from build123d import *

# Parameters (mm, degrees)
F0_R     = 25
F0_W     = 17
F0_H     = 7
F1_DEPTH = 18
F3_D     = 10
F3_DEPTH = 100
F3_TIP   = 3.0043030951
F4_W     = 17
F4_H     = 1
F5_DEPTH = 2
F6_W     = 3.5
F6_H     = 1
F7_DEPTH = 2


with BuildPart() as f1:
    # F0 (on Top) → F1 (new body)
    with BuildSketch(Plane.XY):
        Circle(F0_R)
        Rectangle(F0_W, F0_H, mode=Mode.SUBTRACT)
    extrude(amount=F1_DEPTH)

    # F3 (one way)
    with BuildSketch(Plane(origin=(0, -3.5, 0), x_dir=(-1, 0, 0), z_dir=(0, -1, 0))):
        with Locations((0, 0)):
            Circle(F3_D / 2)
    extrude(amount=-F3_DEPTH, mode=Mode.SUBTRACT)
    with Locations(Plane(origin=(0, -3.5, 0), x_dir=(-1, 0, 0), z_dir=(0, -1, 0))):
        with Locations((0, 0)):
            with Locations((0, 0, -(F3_DEPTH + F3_TIP / 2))):  # 118° drill point
                Cone(0, F3_D / 2, F3_TIP, mode=Mode.SUBTRACT)

    # F4 (on face) → F5 (join)
    with BuildSketch(Plane(origin=(0, -3.5, 0), x_dir=(-1, 0, 0), z_dir=(0, 1, 0))):
        with Locations((0, 0.5)):
            Rectangle(F4_W, F4_H)
    extrude(amount=F5_DEPTH)

    # F6 (on face) → F7 (join)
    with BuildSketch(Plane.XZ.offset(-3.5)):
        with Locations((-6.75, 0.5)):
            Rectangle(F6_W, F6_H)
        with Locations((6.75, 0.5)):
            Rectangle(F6_W, F6_H)
    extrude(amount=F7_DEPTH)


solid = f1.part
Geometry check sheet. Reference: the model listing, model coordinates, mm. A direction names the side the tool comes from. Coordinates: 2 decimals unless noted, no trailing zeros. Order: outer loops, then holes, each group sorted by start corner. A loop starts at its lowest first (then second) coordinate and runs counter-clockwise, first axis right, second up. Notation, with made-up numbers: (51.5, 83) - (62.5, 83) arc R35 ccw to (62.5, 122) - close; hole circle Ø4 at (33.25, -7.75). An arc over 180 degrees is marked (long way). Answer in a Markdown table with one row per item. Add a question column.
1) Gauge pin test, flat ends, axial feed: P1, Ø0.5, axis at x = -1, z = 0.5, coming from the +Y side; P2, Ø0.8, axis at x = 7, z = 0.5, coming from the -Y side; P3, Ø0.8, axis at x = -6, z = 0.5, coming from the -Y side. Record the tip position at first contact, or that the pin passes through.
2) Cross-section at A-A, the plane x = -7. Record the cut outline in (y, z).
3) Material ranges on line 1 along Y through (x, z) = (-8, 8); line 2 along X through (y, z) = (15, 1.75); line 3 along X through (y, z) = (1, 8), recorded low to high. Write a range as [from, to].
4) Cross-section at B-B, the plane y = 0. Record the cut outline in (x, z), then the cut area to 3 significant figures.
5) Cross-section at D-D, the plane x = 0. Record the cut outline in (y, z), then the cut area to 4 significant figures.
6) Release check for a two-part mould opening along Y. For faces 4 (the flat face through (0, -5, 0)), 5 (the flat face through (-7, 3, 1)), 6 (the cylindrical face through (11.5, -22.2, 8.9)) record: +Y half, -Y half, draft (parallel to the pull), parting line (faces both ways), or undercut.
7) Set-up check for faces 1 (the flat face through (0, -3.5, 9)), 2 (the cylindrical face through (0, 14, 5)), 3 (the flat face through (0, -5, 18)): record each of +Z, -Z, +X, -X, +Y, -Y from which the full face is reachable in a straight line by a thin tool's end or side.
8) Cross-section at C-C, the plane z = 11.5. Record the cut outline in (x, y).
Check result:
| question | item | result |
|---|---|---|
| 1 | P1 | stops at y = -1.5 |
| 1 | P2 | stops at y = -24.11 |
| 1 | P3 | stops at y = -24.36 |
| 2 | outline | (-24, 0) - (-1.5, 0) - (-1.5, 1) - (-3.5, 1) - (-3.5, 18) - (-24, 18) - close; (1.5, 0) - (24, 0) - (24, 18) - (3.5, 18) - (3.5, 1) - (1.5, 1) - close |
| 3 | line 1 | y = [-23.69, -3.5], [3.5, 23.69] |
| 3 | line 2 | x = [-20, -4.68], [4.68, 20] |
| 3 | line 3 | x = [-24.98, -8.5], [8.5, 24.98] |
| 4 | outline | (-25, 0) - (-8.5, 0) - (-8.5, 18) - (-25, 18) - close; (8.5, 0) - (25, 0) - (25, 18) - (8.5, 18) - close |
| 4 | area | 594 mm² |
| 5 | outline | (-25, 0) - (-1.5, 0) - (-1.5, 1) - (-3.5, 1) - (-3.5, 18) - (-25, 18) - close; (3.5, 5) - (25, 5) - (25, 18) - (3.5, 18) - close |
| 5 | area | 668.5 mm² |
| 6 | face 4 | draft |
| 6 | face 5 | undercut |
| 6 | face 6 | parting line |
| 7 | face 1 | +Z |
| 7 | face 2 | -Z, +Y |
| 7 | face 3 | +Z, +X, -X, +Y, -Y |
| 8 | outline | circle Ø50 at (0, 0); hole (-8.5, -3.5) - (8.5, -3.5) - (8.5, 3.5) - (-8.5, 3.5) - close |
